Work out the finished part from the listing and answer in its coordinate system (mm). Face numbers are marked on the shaded views. A direction names the side the tool comes from. Round coordinates to 2 decimals unless told otherwise and drop trailing zeros. Write each loop counter-clockwise with the first axis right and the second up, starting at its lowest first coordinate (ties: lowest second). Pieces come first, ordered by that corner, then holes. Notation, with made-up numbers: (-18, -1.5) - (19, -1.5) arc R22 cw to (19, 18.5) - close; hole circle Ø5 at (-4, -20). An arc over 180 degrees is marked (long way). Answer as a JSON object with one key per item and string values.
Autodesk Inventor part; units mm, degrees
ref_plane "YZ Plane" through (0, 0, 0) normal (1, 0, 0) x (0, 1, 0)
ref_plane "XZ Plane" through (0, 0, 0) normal (0, 1, 0) x (-1, 0, 0)
ref_plane "XY Plane" through (0, 0, 0) normal (0, 0, 1) x (1, 0, 0)
sketch "Sketch1" plane through (0, 0, 0) normal (0, 0, 1) x (1, 0, 0)
  line L0 (-8.5, 8.5) -> (8.5, 8.5)
  line L1 (8.5, 8.5) -> (8.5, -8.5)
  line L2 (8.5, -8.5) -> (-8.5, -8.5)
  line L3 (-8.5, -8.5) -> (-8.5, 8.5)
  line L4 (-8.5, 8.5) -> (8.5, -8.5) construction
  line L5 (8.5, 8.5) -> (-8.5, -8.5) construction
  line L6 (5.5, -2.2782) -> (2.2782, -5.5)
  line L7 (2.2782, -5.5) -> (-2.2782, -5.5)
  line L8 (-2.2782, -5.5) -> (-5.5, -2.2782)
  line L9 (-5.5, -2.2782) -> (-5.5, 2.2782)
  line L10 (-5.5, 2.2782) -> (-2.2782, 5.5)
  line L11 (-2.2782, 5.5) -> (2.2782, 5.5)
  line L12 (2.2782, 5.5) -> (5.5, 2.2782)
  line L13 (5.5, 2.2782) -> (5.5, -2.2782)
  line L14 (5.6, -2.3196) -> (2.3196, -5.6)
  line L15 (2.3196, -5.6) -> (-2.3196, -5.6)
  line L16 (-2.3196, -5.6) -> (-5.6, -2.3196)
  line L17 (-5.6, -2.3196) -> (-5.6, 2.3196)
  line L18 (-5.6, 2.3196) -> (-2.3196, 5.6)
  line L19 (-2.3196, 5.6) -> (2.3196, 5.6)
  line L20 (2.3196, 5.6) -> (5.6, 2.3196)
  line L21 (5.6, 2.3196) -> (5.6, -2.3196)
  point P0 (0, 0)
  dimension "d2" = 17
  dimension "d3" = 17
  dimension "d28" = 11
  dimension "d29" = 0.1
extrude "Extrusion1" add sketch "Sketch1" along normal blind 30 contours L0 L1 L2 L3 | L6 L7 L8 L9 L10 L11 L12 L13 | L14 L15 L16 L17 L18 L19 L20 L21
extrude "Extrusion2" cut sketch "Sketch1" along normal blind 15 contours L6 L7 L8 L9 L10 L11 L12 L13 | L14 L15 L16 L17 L18 L19 L20 L21
sketch "Sketch2" plane through (0, 0, 30) normal (0, 0, 1) x (1, 0, 0)
  circle A0 centre (0, 0) radius 6.425
  dimension "d8" = 12.85
extrude "Extrusion3" cut sketch "Sketch2" against normal blind 15
sketch "Sketch3" plane through (-8.5, 8.5, 0) normal (0, 1, 0) x (1, 0, 0)
  line L0 (17, 0) -> (0, 0)
  line L1 (0, 0) -> (0, -30)
  line L2 (17, -30) -> (0, -30)
  line L3 (17, 0) -> (17, -30)
  line L4 (0, 0) -> (0, -30) construction
  line L5 (0, -30) -> (17, -15)
  line L6 (17, 0) -> (17, -30) construction
  circle A0 centre (8.5, -22.5) radius 6.425
  line L7 (17, -30) -> (0, -15)
  line L8 (0, 0) -> (0, -30) construction
  point P0 (8.5, 0)
  dimension "d11" = 12.85
extrude "Extrusion4" cut sketch "Sketch3" against normal through all contours A0 L7 L5 | L5 L7 A0 | L7 L5 A0 | A0 L5 L7
sketch "Sketch4" plane through (8.5, -8.5, 0) normal (1, 0, 0) x (0, 0, -1)
  line L0 (0, 17) -> (-30, 17) construction
  line L1 (-15, 17) -> (-15, 0) construction
  line L2 (0, 0) -> (-30, 0) construction
  line L3 (-30, 17) -> (-30, 0) construction
  line L4 (-30, 17) -> (-15, 0) construction
  line L5 (-15, 17) -> (-30, 0) construction
  circle A0 centre (-22.5, 8.5) radius 2.8
  circle A1 centre (-22.5, 8.5) radius 5
  point P0 (0, 8.5)
  dimension "d14" = 5.6
  dimension "d15" = 10
ref_plane "Work Plane1" through (-8.5, 0, 0) normal (0, -1, 0) x (1, 0, 0)
sketch "Sketch5" plane through (-8.5, 0, 0) normal (0, -1, 0) x (1, 0, 0)
  line L0 (17, 0) -> (17, 30) construction
  line L1 (0, 0) -> (0, 30) construction
  line L2 (17, 0) -> (0, 0) construction
  line L3 (17, 30) -> (0, 30) construction
  point P0 (8.5, 0)
  point P1 (17, 22.5)
  point P2 (0, 7.5)
  dimension "d23" = 7.5
  dimension "d24" = 7.5
extrude "Extrusion5" add sketch "Sketch4" along normal blind 3
extrude "Extrusion6" cut sketch "Sketch4" against normal blind 5 contours A0
pattern_sketch "Sketch Driven Pattern1" of "Extrusion6", "Extrusion5" from (8.5, 0, 22.5) facing (1, 0, 0) copies at (-8.5, 0, 7.5) facing (-1, 0, 0)
chamfer "Chamfer2" distance 3 angle 45 2 edges at (8.5, 0, 27.5) (-8.5, 0, 2.5)
equation "\"d2\" = d3"
properties part number "waxing_station"
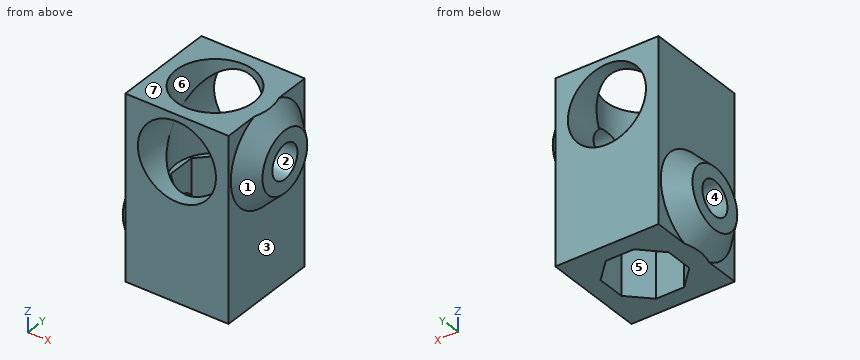
Item 1: For the marked faces 5, 6 and 7, determine the directions among +Z, -Z, +X, -X, +Y, -Y from which every point of the face is accessible in a straight line to the end or side of a thin tool.
Results found:
{"face 5": "+Z, -Z", "face 6": "+Z", "face 7": "+Z, +X, -X, +Y, -Y"}
Item 2: A cutting plane is placed at C-C (x = 4.5). Write down the section's boundary in (y, z).
Results found:
{"outline": "(-8.5, 0) - (-3.42, 0) - (-3.42, 15) - (-4.59, 15) - (-4.59, 17.91) - (-8.5, 17.91) - close; (-8.5, 27.09) - (-4.59, 27.09) - (-4.59, 30) - (-8.5, 30) - close; (3.42, 0) - (8.5, 0) - (8.5, 17.91) - (4.59, 17.91) - (4.59, 15) - (3.42, 15) - close; (4.59, 27.09) - (8.5, 27.09) - (8.5, 30) - (4.59, 30) - close"}
Item 3: Consider line 1 along Z through (x, y) = (0.25, 6.75); line 2 along Y through (x, z) = (0.75, 12); line 3 along Y through (x, z) = (-4.5, 2). Determine where each line is inside the solid, lowest interval first.
Results found:
{"line 1": "0 to 16.08, 28.92 to 30", "line 2": "-8.5 to -5.6, 5.6 to 8.5", "line 3": "-8.5 to -3.42, 3.42 to 8.5"}
Item 4: A cutting plane is placed at B-B (x = 10). Write down the section's boundary in (y, z), and give its area (3 significant figures).
Results found:
{"outline": "circle Ø13 at (0, 22.5); hole circle Ø5.6 at (0, 22.5)", "area": "108 mm²"}
Item 5: Determine the mould class of the marked faces 1, 2, 3 and 4 for opening direction Z: pulls with the +Z half, pulls with the -Z half, needs draft (parallel to the pull), parting line crosses it, or undercut.
Results found:
{"face 1": "parting line crosses it", "face 2": "undercut", "face 3": "needs draft", "face 4": "undercut"}
Item 6: A cutting plane is placed at D-D (y = 0.5). Give the number of separate pieces and of enclosed holes in the cut face, and give its area (3 significant figures).
Results found:
{"separate pieces": "4", "enclosed holes": "0", "area": "167 mm²"}
Item 7: Each of these flat-tipped pins is pushed along its axis until it touches: P1, Ø4, axis at y = -1, z = 15.5, coming from the -X side; P2, Ø10, axis at x = 0.5, y = 5.5, coming from the +Z side; P3, Ø1.4, axis at y = -1, z = 2.5, coming from the +X side; P4, Ø7.5, axis at y = 0, z = 22.5, coming from the -X side. Where does it stop, or does it pass through?
Results found:
{"P1": "x = -10.44", "P2": "z = 30", "P3": "x = 8.5", "P4": "x = -8.5"}
Item 8: A cutting plane is placed at A-A (x = 0). Write down the section's boundary in (y, z) (3 decimals).
Results found:
{"outline": "(-8.5, 0) - (-5.6, 0) - (-5.6, 15) - (-6.425, 15) - (-6.425, 16.075) - (-8.5, 16.075) - close; (-8.5, 28.925) - (-6.425, 28.925) - (-6.425, 30) - (-8.5, 30) - close; (5.6, 0) - (8.5, 0) - (8.5, 16.075) - (6.425, 16.075) - (6.425, 15) - (5.6, 15) - close; (6.425, 28.925) - (8.5, 28.925) - (8.5, 30) - (6.425, 30) - close"}
